Autodesk Inventor part; units mm, degrees
ref_plane "YZ Plane" through (0, 0, 0) normal (1, 0, 0) x (0, 1, 0)
ref_plane "XZ Plane" through (0, 0, 0) normal (0, 1, 0) x (-1, 0, 0)
ref_plane "XY Plane" through (0, 0, 0) normal (0, 0, 1) x (1, 0, 0)
sketch "Sketch7" plane through (0, 0, 0) normal (0, 0, 1) x (1, 0, 0)
  line L0 (0, 0) -> (300, 0)
  line L1 (300, 0) -> (300, 60)
  line L2 (300, 60) -> (0, 60)
  line L3 (0, 60) -> (0, 0)
  line L4 (50, 13) -> (250, 13)
  line L5 (250, 13) -> (250, 10)
  line L6 (250, 10) -> (50, 10)
  line L7 (50, 10) -> (50, 13)
  line L8 (150, 13) -> (150, 10) construction
  line L9 (20, 50) -> (40, 50)
  line L10 (40, 50) -> (40, 10)
  line L11 (40, 10) -> (20, 10)
  line L12 (20, 10) -> (20, 50)
  line L13 (260, 50) -> (280, 50)
  line L14 (280, 50) -> (280, 10)
  line L15 (280, 10) -> (260, 10)
  line L16 (260, 10) -> (260, 50)
  line L17 (50, 47) -> (250, 47)
  line L18 (250, 47) -> (250, 50)
  line L19 (250, 50) -> (50, 50)
  line L20 (50, 50) -> (50, 47)
  point P0 (50, 48.5)
  point P1 (50, 11.5)
  dimension "d152" = 300
  dimension "d153" = 60
  dimension "d154" = 200
  dimension "d158" = 150
  dimension "d159" = 3
  dimension "d160" = 10
  dimension "d161" = 40
  dimension "d162" = 20
  dimension "d163" = 20
  dimension "d164" = 20
  dimension "d165" = 10
  dimension "d166" = 10
  dimension "d168" = 10
extrude "Extrusion7" add sketch "Sketch7" along normal blind 3.3
fillet "Fillet1" radius 6 4 edges at (0, 60, 1.65) (0, 0, 1.65) (300, 60, 1.65) (300, 0, 1.65)
sketch "Sketch9" plane through (0, 0, 3.3) normal (0, 0, 1) x (1, 0, 0)
  arc A0 (294, 0) -> (300, 6) centre (294, 6) ccw
  line L0 (300, 6) -> (300, 54)
  arc A1 (300, 54) -> (294, 60) centre (294, 54) ccw
  line L1 (294, 60) -> (6, 60)
  arc A2 (6, 60) -> (0, 54) centre (6, 54) ccw
  line L2 (0, 54) -> (0, 6)
  arc A3 (0, 6) -> (6, 0) centre (6, 6) ccw
  line L3 (6, 0) -> (294, 0)
  line L4 (280, 50) -> (280, 10)
  line L5 (280, 10) -> (260, 10)
  line L6 (260, 10) -> (260, 50)
  line L7 (260, 50) -> (280, 50)
  line L8 (40, 50) -> (40, 10)
  line L9 (40, 10) -> (20, 10)
  line L10 (20, 10) -> (20, 50)
  line L11 (20, 50) -> (40, 50)
  line L12 (50, 47) -> (50, 50)
  line L13 (50, 50) -> (250, 50)
  line L14 (250, 50) -> (250, 47)
  line L15 (250, 47) -> (50, 47)
  line L16 (250, 13) -> (250, 10)
  line L17 (250, 10) -> (50, 10)
  line L18 (50, 10) -> (50, 13)
  line L19 (50, 13) -> (250, 13)
  line L20 (50, 18) -> (74, 42)
  line L21 (74, 42) -> (84, 42)
  line L22 (84, 42) -> (60, 18)
  line L23 (60, 18) -> (50, 18)
  point P0 (0, 0)
  dimension "d172" = 45
  dimension "d173" = 10
  dimension "d175" = 5
  dimension "d182" = 5
extrude "Extrusion8" cut sketch "Sketch9" against normal blind 3.3 contours L20 L21 L22 L23
pattern_linear "Rectangular Pattern1" count 7 spacing 27 along (1, 0, 0) of "Extrusion8"
sketch "Sketch10" plane through (0, 0, 3.3) normal (0, 0, 1) x (1, 0, 0)
  line L0 (20, 10) -> (20, 50)
  line L1 (20, 50) -> (40, 50)
  line L2 (40, 50) -> (40, 10)
  line L3 (40, 10) -> (20, 10)
  circle A0 centre (25, 54.75) radius 1
  circle A1 centre (35, 54.75) radius 1
  circle A2 centre (25, 5.25) radius 1
  circle A3 centre (35, 5.25) radius 1
  line L4 (260, 10) -> (260, 50)
  line L5 (280, 50) -> (280, 10)
  line L6 (260, 50) -> (280, 50)
  line L7 (280, 10) -> (260, 10)
  circle A4 centre (265, 54.75) radius 1
  circle A5 centre (275, 54.75) radius 1
  circle A6 centre (265, 5.25) radius 1
  circle A7 centre (275, 5.25) radius 1
  point P0 (0, 0)
  dimension "d183" = 2
  dimension "d184" = 5
  dimension "d185" = 10
  dimension "d186" = 5
  dimension "d187" = 10
  dimension "d188" = 4.75
  dimension "d189" = 4.75
  dimension "d192" = 2
  dimension "d194" = 10
  dimension "d196" = 10
  dimension "d202" = 5
extrude "Extrusion9" cut sketch "Sketch10" against normal blind 10 contours A0 | A1 | A2 | A3 | A4 | A5 | A6 | A7
equation "\"soporte\" = 60"
equation "\"largo_base\" = 200"
properties part number "Cuerpo - LateralPrueba" material "ABS Plastic"
Here's how the part is built. I have some questions about the finished solid (model axes, mm). A direction names the side the tool comes from. Coordinates: 2 decimals unless noted, no trailing zeros. Write each loop counter-clockwise with the first axis right and the second up, starting at its lowest first coordinate (ties: lowest second). Pieces come first, ordered by that corner, then holes. Notation, with made-up numbers: (74.5, -14.5) - (113.5, -14.5) arc R23 ccw to (113.5, 9.5) - close; hole circle Ø11 at (52.5, 14.25). An arc over 180 degrees is marked (long way). Use one line per item in the form item = value.
1) I need wall thicknesses on line 1 (Y direction, x = 35, z = 2.5); line 2 (X direction, y = 44.5, z = 2.3); line 3 (X direction, y = 12.5, z = 1.25). Which ranges of each line are inside material? Lowest first, please.
Solved:
line_1 = 0 to 4.25, 6.25 to 10, 50 to 53.75, 55.75 to 60
line_2 = 0 to 20, 40 to 260, 280 to 300
line_3 = 0 to 20, 40 to 50, 250 to 260, 280 to 300
2) Suppose I cut it at A-A, the plane x = 224.5. Write out the boundary of the cut face in (y, z).
Solved:
outline = (0, 0) - (10, 0) - (10, 3.3) - (0, 3.3) - close; (13, 0) - (20.5, 0) - (20.5, 3.3) - (13, 3.3) - close; (30.5, 0) - (47, 0) - (47, 3.3) - (30.5, 3.3) - close; (50, 0) - (60, 0) - (60, 3.3) - (50, 3.3) - close
3) On a 3-axis mill with a long thin cutter (end or side, diameter ignored), from which of +Z, -Z, +X, -X, +Y, -Y can I reach the whole of each face in a straight line? I mean faces 4 (the flat face through (170, 30, 2)), 5 (the flat face through (148, 37, 3.3)). Say none if no direction works.
Solved:
face_4 = +Z, -Z
face_5 = +Z, +X, -X, +Y, -Y
4) Thinking about a two-plate mould opening in Y: for faces 1 (the cylindrical face through (1.711, 1.804, 1.673)), 2 (the cylindrical face through (298.289, 58.196, 1.673)), 3 (the flat face through (72, 30, 2)), which applies, released by +Y, released by -Y, zero draft, split by the parting line, or undercut?
Solved:
face_1 = released by -Y
face_2 = released by +Y
face_3 = undercut
5) I'm going to push flat-ended pins straight in: P1, Ø2, axis at x = 253, y = 12, coming from the -Z side; P2, Ø1.2, axis at x = 275, y = 54.75, coming from the -Z side. Where does each tip first touch, or does it pass through?
Solved:
P1 = 0
P2 = through
6) Suppose I cut it at B-B, the plane y = 38. Give the number of separate pieces and of enclosed holes in the cut face, plus the area to 3 significant figures.
Solved:
separate_pieces = 10
enclosed_holes = 0
area = 627 mm2
